from build123d import *

# Parameters (mm, degrees)
F1_DEPTH = 127
F2_DEPTH = 19.05
F4_DEPTH = 38.1


# Not quite as in the source:
# - a pattern or mirror of a feature is missing from the dataset's text; its kind, count and spacing are read off the source's solid


with BuildPart() as f1:
    # F0 (on Front) → F1 (new body, symmetric)
    with BuildSketch(Plane.XZ):
        Polygon((0, 254), (0, 0), (254, 0), (254, 38.1), (177.8, 38.1), (38.1, 38.1), (38.1, 139.7), (38.1, 222.25), align=None)
    extrude(amount=F1_DEPTH, both=True)

    # F0 (on Front) → F2 (join, symmetric)
    with BuildSketch(Plane.XZ):
        Polygon((38.1, 38.1), (177.8, 38.1), (88.9, 139.7), (38.1, 139.7), align=None)
    extrude(amount=F2_DEPTH, both=True)

    # F3 (on face) → F4 (join)
    with BuildSketch(Plane.XZ.offset(127)):
        Polygon((254, 38.1), (38.1, 114.3), (38.1, 38.1), align=None)
    f4 = extrude(amount=-F4_DEPTH)

    # F4_copies: F4 across plane
    add(f4.mirror(Plane.ZX))


solid = f1.part
Here's how the part is built. I have some questions about the finished solid (model axes, mm). A direction names the side the tool comes from. Round coordinates to 2 decimals unless told otherwise and drop trailing zeros. Order: outer loops, then holes, each group sorted by start corner. A loop starts at its lowest first (then second) coordinate and runs counter-clockwise, first axis right, second up. Notation, with made-up numbers: M 0,18.5 L 47,18.5 A20 ccw 47,39.5 Z; hole C 56,-6.75 d5. An arc over 180 degrees is marked long. Return JSON: item names as keys, results as strings. Group by question number.
1. If we section it at C-C on z = 70: List the corners of the cut face in (x, y) for me, then the cut area to 3 significant figures.
2. On a 3-axis mill with a long thin cutter (end or side, diameter ignored), from which of +Z, -Z, +X, -X, +Y, -Y can I reach the whole of each face in a straight line? I mean faces 1 (the face through (91, 19.05, 78)), 2 (the face through (147.561, 108.217, 75.667)), 3 (the face through (147.561, -108.217, 75.667)). Say none if no direction works.
3. If we mould it in two halves opening along Y, with no side actions, what happens to faces 4 (the face through (64, 0, 139.7)), 5 (the face through (91, -19.05, 78)), 6 (the face through (97, 127, 72))? For each: pulls with the +Y half, pulls with the -Y half, needs draft (parallel to the pull), parting line crosses it, or undercut.
4. Please list where these lines run through material, in increasing order: probe 1 along Y at (x, z) = (195, 46); probe 2 along X at (y, z) = (56, 145); probe 3 along Z at (x, y) = (52, -11).
5. If we section it at A-A on y = 7: List the corners of the cut face in (x, z) for me.
6. If we section it at D-D on y = 52.5: List the corners of the cut face in (x, z) for me, then the cut area to 3 significant figures.
7. If we section it at B-B on x = 193.5: List the corners of the cut face in (y, z) for me.
8. I'm going to push flat-ended pins straight in: pin 1 Ø3 at (x, z) = (109, 104.5) entering from +Y; pin 2 Ø4 at (y, z) = (48, 176.5) entering from -X; pin 3 Ø1.5 at (y, z) = (19, 214.5) entering from +X; pin 4 Ø11.5 at (x, y) = (57, -5.5) entering from +Z. Where does each tip first touch, or does it pass through?
Reply:
{
 "1": {"outline": "M 0,-127 L 163.62,-127 L 163.62,-88.9 L 38.1,-88.9 L 38.1,-19.05 L 149.89,-19.05 L 149.89,19.05 L 38.1,19.05 L 38.1,88.9 L 163.62,88.9 L 163.62,127 L 0,127 Z", "area": "23,500 mm^2"},
 "2": {"face 1": "+Z, +X", "face 2": "+Z, +X, +Y", "face 3": "+Z, +X, -Y"},
 "3": {"face 4": "needs draft", "face 5": "undercut", "face 6": "pulls with the +Y half"},
 "4": {"probe 1": "-127 to -88.9, 88.9 to 127", "probe 2": "0 to 38.1", "probe 3": "0 to 139.7"},
 "5": {"outline": "M 0,0 L 254,0 L 254,38.1 L 177.8,38.1 L 88.9,139.7 L 38.1,139.7 L 38.1,222.25 L 0,254 Z"},
 "6": {"outline": "M 0,0 L 254,0 L 254,38.1 L 38.1,38.1 L 38.1,222.25 L 0,254 Z", "area": "17,300 mm^2"},
 "7": {"outline": "M -127,0 L 127,0 L 127,59.45 L 88.9,59.45 L 88.9,38.1 L -88.9,38.1 L -88.9,59.45 L -127,59.45 Z"},
 "8": {"pin 1": "y = 19.05", "pin 2": "x = 0", "pin 3": "x = 38.1", "pin 4": "z = 139.7"}
}
